Solid Edge part; units mm, degrees
sketch "Sketch1" plane through (0, 0, 0) normal (0, -1, 0) x (1, 0, 0)
  line L0 (0, 15) -> (0, 41)
  line L1 (0, 41) -> (8, 41)
  line L2 (8, 41) -> (8, 23)
  line L3 (8, 23) -> (28, 23)
  line L4 (28, 23) -> (28, 15)
  line L5 (28, 15) -> (0, 15)
  dimension "D1" = 28
  dimension "D2" = 8
revolve "RevolvedProtrusion1" add sketch "Sketch1" angle 360 about axis through (0, 0, 0) along (1, 0, 0)
hole "Hole1" at (8, 0, 32) direction (-1, 0, 0) diameter 8 end up to next
pattern_circular "Pattern2" count 4 over 360 about axis through (8, 0, 0) along (-1, 0, 0) of "Hole1"
sketch "Sketch2" plane through (28, 0, 0) normal (1, 0, 0) x (0, 1, 0)
  line L0 (7.3941, 13.051) -> (10.2225, 15.8794)
  line L1 (10.2225, 15.8794) -> (15.8794, 10.2225)
  line L2 (15.8794, 10.2225) -> (13.051, 7.3941)
  line L3 (13.051, 7.3941) -> (7.3941, 13.051)
  dimension "D1" = 10.2225
  dimension "D2" = 15.8794
extrude "Cutout1" cut sketch "Sketch2" against normal up to vertex (20 mm away)
sketch "Sketch3" plane through (0, 0, 0) normal (0, 1, 0) x (-1, 0, 0)
  line L0 (0, 15) -> (1.2473, 15)
  line L1 (1.2473, 15) -> (1.2473, 16.2473)
  line L2 (1.2473, 16.2473) -> (0, 16.2473)
  line L3 (0, 16.2473) -> (0, 15)
  dimension "D1" = 1.2473
revolve "RevolvedProtrusion2" add sketch "Sketch3" angle 360 about axis through (0, 0, 0) along (1, 0, 0)
hole "Hole2" at (21, 13.051, 13.051) direction (0, 0.7071068, 0.7071068) diameter 5 end up to next
properties material "Steel"
Input: part model. Units: mm. Frame: model coordinates. A direction names the side the tool comes from. Give positions to 0.01 mm unless a question says otherwise; leave off trailing zeros. Order: outer loops, then holes, each group sorted by start corner. A loop starts at its lowest first (then second) coordinate and runs counter-clockwise, first axis right, second up.
1. Draft query along Z for faces 4 (the face through (4, 40, -9)), 5 (the face through (28, 15, 5)), 6 (the face through (4.1, 2.4, -35.2)). Return one class per face: released by +Z, released by -Z, zero draft, split by the parting line, or undercut.
Computed:
face 4: split by the parting line
face 5: zero draft
face 6: undercut
2. Cut plane D-D (z = -32). Return loops of the section in (x, y), and give its area (3 significant figures).
Computed:
outline: (0, -25.63) - (8, -25.63) - (8, -4) - (0, -4) - close; (0, 4) - (8, 4) - (8, 25.63) - (0, 25.63) - close
area: 346 mm2
3. Pin query (flat end, axial travel): pin 1 Ø5 at (x, y) = (13.5, -2.5) entering from +Z; pin 2 Ø1.5 at (y, z) = (27, -26.5) entering from -X; pin 3 Ø12 at (x, z) = (10.5, -23.5) entering from +Y; pin 4 Ø24.5 at (y, z) = (18, -12.5) entering from -X. Return the tip coordinate at first contact, or that it passes through.
Computed:
pin 1: stops at z = 23
pin 2: stops at x = 0
pin 3: stops at y = 36.82
pin 4: stops at x = -1.25
4. Cut plane C-C (x = 19.75). Return loops of the section in (y, z), and give its area (3 significant figures).
Computed:
outline: (7.39, 13.05) - (10.22, 15.88) - (11.52, 14.58) - (14.66, 17.72) arc R23 ccw (long way) to (17.72, 14.66) - (14.58, 11.52) - (15.88, 10.22) - (13.05, 7.39) arc R15 cw (long way) to start
area: 906 mm2
5. Set-up query: faces 1 (the face through (23.479, 14.405, 14.865)), 2 (the face through (0, -1, 18)), 3 (the face through (18.14, 8.789, 14.445)). Return all of +Z, -Z, +X, -X, +Y, -Y with unobstructed straight access to the full face (end or side cutting, diameter ignored); none if empty.
Computed:
face 1: none
face 2: -X
face 3: +X
6. Cut plane A-A (y = 0). Return loops of the section in (x, z).
Computed:
outline: (-1.25, -16.25) - (0, -16.25) - (0, -28) - (8, -28) - (8, -23) - (28, -23) - (28, -15) - (-1.25, -15) - close; (-1.25, 15) - (28, 15) - (28, 23) - (8, 23) - (8, 28) - (0, 28) - (0, 16.25) - (-1.25, 16.25) - close; (0, -41) - (8, -41) - (8, -36) - (0, -36) - close; (0, 36) - (8, 36) - (8, 41) - (0, 41) - close
7. Line query: probe 1 along Z at (x, y) = (5, 0); probe 2 along Z at (x, y) = (10.5, 0). Output: solid intervals per line, ascending.
Computed:
probe 1: z = -41 to -36, -28 to -15, 15 to 28, 36 to 41
probe 2: z = -23 to -15, 15 to 23
